Check sheet for the modelled part. Datum: model origin and axes. Units: mm. A direction names the side the tool comes from. Round coordinates to 2 decimals unless told otherwise and drop trailing zeros. Order: outer loops, then holes, each group sorted by start corner. A loop starts at its lowest first (then second) coordinate and runs counter-clockwise, first axis right, second up. Notation, with made-up numbers: (20.5, -26.75) -> (71.5, -26.75) arc R15 ccw to (71.5, -3.75) -> close; hole circle Ø7 at (-9, -8.75). An arc over 180 degrees is marked (long way). Answer in a Markdown table with one row per item.
Autodesk Inventor part; units mm, degrees
ref_plane "Work Plane1" through (29, 0, 0) normal (0, -1, 0) x (1, 0, 0)
ref_plane "YZ Plane" through (0, 0, 0) normal (1, 0, 0) x (0, 1, 0)
ref_plane "XZ Plane" through (0, 0, 0) normal (0, 1, 0) x (-1, 0, 0)
sketch "Sketch1" plane through (0, 0, 0) normal (0, 0, 1) x (1, 0, 0)
  line L0 (-0.8667, 0) -> (40, 0)
  line L1 (40, 0) -> (40, 1.5)
  line L2 (40, 1.5) -> (33.25, 1.5)
  line L3 (33.25, 1.5) -> (32.9432, 1.5)
  line L4 (32.9432, 1.5) -> (0, 1.5)
  line L5 (0, 1.5) -> (0, 2.75)
  line L6 (0, 2.75) -> (-3, 2.75)
  line L7 (-3, 2.75) -> (-3, 1.4434)
  line L8 (-3, 1.4434) -> (-1.7, 1.4434)
  line L9 (-1.7, 1.4434) -> (-0.8667, 0)
  line L10 (-11.6, 0) -> (48.6, 0)
  line L11 (0, -0.55) -> (0, 3.3)
  line L12 (33.25, 1.5) -> (0, 1.5) construction
  dimension "d1" = 6.75
  dimension "d2" = 0.3068
  dimension "d3" = 3
  dimension "d4" = 1.3
  dimension "d5" = 60
  dimension "d6" = 3
  dimension "d7" = 3
  dimension "d8" = 2.8868
  dimension "d9" = 5.5
  dimension "d26" = 40
revolve "Body" add sketch "Sketch1" angle 360 about axis through (-0.8667, 0, 0) along (1, 0, 0)
sketch "Sketch2" plane through (-3, 0, 0) normal (-1, 0, 0) x (0, 0, 1)
  circle A0 centre (0, 0) radius 1.4434
  line L0 (0, -3.85) -> (0, 3.85)
  line L1 (-3.85, 0) -> (3.85, 0)
  line L2 (1.4434, 0) -> (0.7217, -1.25)
  line L3 (0.7217, -1.25) -> (-0.7217, -1.25)
  line L4 (-0.7217, -1.25) -> (-1.4434, 0)
  line L5 (-1.4434, 0) -> (-0.7217, 1.25)
  line L6 (-0.7217, 1.25) -> (0.7217, 1.25)
  line L7 (0.7217, 1.25) -> (1.4434, 0)
extrude "Slot" add sketch "Sketch2" against normal up to next contours L7 A0 | A0 L2 | L6 L0 A0 | A0 L0 L3 | L0 L6 A0 | A0 L3 L0 | L4 A0 | A0 L5
fillet "Fillet1" radius 0.3 1 edges at (-3, -2.75, 0)
thread "Thread"
chamfer "Chamfer1" distance 0.3067 distance2 0.3067 1 edges at (40, -1.5, 0) measured on face at (40, -0.1088, 0.5667)
ref_plane "Work Plane1" through (29, 0, 0) normal (0, -1, 0) x (1, 0, 0)
fillet "Fillet2" radius 0.1 1 edges at (0, -1.5, 0)
equation "\"d1\" = GEL"
equation "\"d3\" = KOH"
equation "\"d4\" = INTI"
equation "\"d6\" = GD"
equation "\"d7\" = BDM"
equation "\"d8\" = 1.1547 * SW"
equation "\"d9\" = KOD"
equation "\"d30\" = R"
equation "\"d17\" = RR"
equation "\"d13\" = GEL"
equation "\"d15\" = -0.5 * SPD + 0.5 * GD"
equation "\"d16\" = GUL"
equation "\"GD\" = NND"
equation "\"NLG\" = 8"
equation "\"GEL\" = 6.75"
equation "\"KOD\" = 5.5"
equation "\"KOH\" = NND"
equation "\"INTI\" = 1.3"
equation "\"GAL\" = 0.61345 * PTC"
equation "\"GUL\" = 0.61345 * PTC"
equation "\"BDM\" = NND"
equation "\"SW\" = 2.5"
equation "\"RR\" = 0.1 * NND"
equation "\"SPD\" = NND - 1.2269 * PTC"
equation "\"R\" = 0.1"
equation "\"PHH\" = 0.13"
equation "\"GD1\" = THREADDIA - 1.2269 * PTC"
equation "\"THREADDIA\" = 3"
equation "\"FAWI\" = 45deg"
equation "\"PTC\" = 0.5"
equation "\"KOH1\" = 2.7"
equation "\"NND\" = 3"
equation "\"TOA\" = 30deg"
equation "\"E0\" = 1.155 * SW"
properties part number "AS 1420 - 1973 - M3 x 8" material "Steel, Mild"
(1) Scan lines: probe 1 along X at (y, z) = (1.05, -2); probe 2 along Z at (x, y) = (21, 0.4); probe 3 along Z at (x, y) = (2, -0.25). Record each from-to range of solid material in increasing order. Write a range as from..to.
Solutions:
| item | result |
|---|---|
| probe 1 | -3..0 |
| probe 2 | -1.45..1.45 |
| probe 3 | -1.48..1.48 |
(2) Draft check along Y on faces 4 (the cylindrical face through (-1.369, -0.596, 2.685)), 5 (the flat face through (40, 0, 0)), 6 (the flat face through (-2.3, -0.63, -1.08)). Enter one of: pulls with the +Y half, pulls with the -Y half, needs draft (parallel to the pull), parting line crosses it, or undercut.
Solutions:
| item | result |
|---|---|
| face 4 | parting line crosses it |
| face 5 | needs draft |
| face 6 | undercut |
(3) Section check A-A on x = 14.5. Record the boundary of the cut face in (y, z), plus the area to 3 significant figures.
Solutions:
| item | result |
|---|---|
| outline | circle Ø3 at (0, 0) |
| area | 7.07 mm^2 |
(4) Tool access check on faces 1 (the flat face through (-2.304, -0.616, 1.088)), 2 (the flat face through (0, 2, 0)), 3 (the flat face through (-3, -1.1, 1.1)). Record the directions out of +Z, -Z, +X, -X, +Y, -Y that give a thin tool (end or side, any length) a straight path to the whole face; none if there is none.
Solutions:
| item | result |
|---|---|
| face 1 | -X |
| face 2 | +X |
| face 3 | +Z, -Z, -X, +Y, -Y |
(5) Depth check by flat-ended pin: pin 1 Ø1.6 at (y, z) = (-1.5, 1) entering from +X; pin 2 Ø1.5 at (x, y) = (29.5, 2) entering from +Z; pin 3 Ø2 at (x, y) = (7, 0) entering from -Z; pin 4 Ø2 at (x, z) = (8.5, 1) entering from +Y. Enter the tip coordinate at first touch or a pass-through.
Solutions:
| item | result |
|---|---|
| pin 1 | x = 40 |
| pin 2 | z = 0.83 |
| pin 3 | z = -1.5 |
| pin 4 | y = 1.5 |
